Input: part model. Units: mm. Frame: model coordinates. Face numbers are marked on the shaded views. A direction names the side the tool comes from. Round coordinates to 2 decimals unless told otherwise and drop trailing zeros. Loops run counter-clockwise (first coordinate to the right, second up) from the corner with the lowest first, then second, coordinate; pieces in that order, holes last. Notation, with made-up numbers: M -2.75,-13 L 43.25,-13 A9 cw 43.25,-8 Z; hole C -29.5,45 d5. An arc over 180 degrees is marked long. Put each result on its own line as item: value. Start each with the question number.
1) Section A-A on x = 38.1. Output: boundary loops of the cut face in (y, z) (1 decimal), plus the area to 3 significant figures.
2) Section C-C on z = 34.5. Output: boundary loops of the cut face in (x, y).
3) Pin query (flat end, axial travel): pin 1 (8.5 mm diameter, centred on x = 55.17, y = 66.7, fed in from +Z); pin 2 (1.5 mm diameter, centred on x = 41, z = 29, fed in from +Y). Return the tip coordinate at first contact, or that it passes through.
4) Reachability of the marked faces 1 and 2 from +Z, -Z, +X, -X, +Y, -Y: full face, straight path, thin tool, end or side. Return the list, or none.
5) Section B-B on y = 17.5. Output: boundary loops of the cut face in (x, z).
6) Line query: probe 1 along Z at (x, y) = (38.1, 3.5) (1 decimal); probe 2 along Y at (x, z) = (15, 57); probe 3 along Z at (x, y) = (49.5, 26). Output: solid intervals per line, ascending.
from build123d import *

# Parameters (mm, degrees)
SKETCH1_W           = 76.2
SKETCH1_H           = 73.0504
SKETCH1_R           = 2.6416
BOSS_EXTRUDE1_DEPTH = 6.604
SKETCH2_W           = 76.2
SKETCH2_H           = 6.604
BOSS_EXTRUDE2_DEPTH = 98.425
SKETCH3_R           = 11.43
SKETCH3_R_2         = 3.175
CUT_EXTRUDE1_DEPTH  = 76.2


with BuildPart() as part:
    # Sketch1 → Boss-Extrude1 (new body)
    with BuildSketch(Plane.XY):
        with Locations((38.1, 36.5252)):
            Rectangle(SKETCH1_W, SKETCH1_H)
        with Locations((21.0312, 66.7004)):
            Circle(SKETCH1_R, mode=Mode.SUBTRACT)
        with Locations((55.1688, 66.7004)):
            Circle(SKETCH1_R, mode=Mode.SUBTRACT)
    extrude(amount=-BOSS_EXTRUDE1_DEPTH)

    # Sketch2 → Boss-Extrude2 (add)
    with BuildSketch(Plane.XY):
        with Locations((38.1, 3.302)):
            Rectangle(SKETCH2_W, SKETCH2_H)
    extrude(amount=BOSS_EXTRUDE2_DEPTH)

    # Sketch3 → Cut-Extrude1 (cut)
    with BuildSketch(Plane(origin=(0, 6.604, 0), x_dir=(1, 0, 0), z_dir=(0, 1, 0))):
        with Locations((38.1, -52.3875)):
            Circle(SKETCH3_R)
        with Locations((38.1, -77.3875)):
            Circle(SKETCH3_R_2)
        with Locations((16.449364905, -39.8875)):
            Circle(SKETCH3_R_2)
        with Locations((59.750635095, -39.8875)):
            Circle(SKETCH3_R_2)
    extrude(amount=-CUT_EXTRUDE1_DEPTH, mode=Mode.SUBTRACT)


solid = part.part
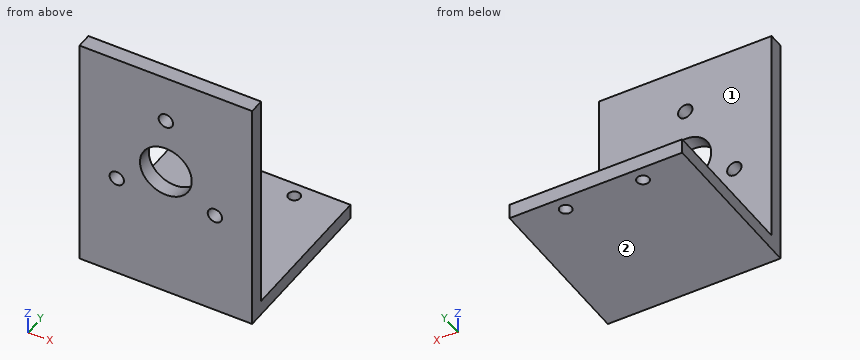
Geometry results:
1. outline: M 0,-6.6 L 73.1,-6.6 L 73.1,0 L 6.6,0 L 6.6,41 L 0,41 Z; M 0,63.8 L 6.6,63.8 L 6.6,74.2 L 0,74.2 Z; M 0,80.6 L 6.6,80.6 L 6.6,98.4 L 0,98.4 Z
1. area: 940 mm²
2. outline: M 0,0 L 76.2,0 L 76.2,6.6 L 0,6.6 Z
3. pin 1: stops at z = 0
3. pin 2: stops at y = 6.6
4. face 1: +Z, +X, -X, +Y
4. face 2: -Z, +X, -X, +Y, -Y
5. outline: M 0,-6.6 L 76.2,-6.6 L 76.2,0 L 0,0 Z
6. probe 1: z = -6.6 to 41, 63.8 to 74.2, 80.6 to 98.4
6. probe 2: y = 0 to 6.6
6. probe 3: z = -6.6 to 0
